Verification items for the finished model (mm, model axes). Round coordinates to 2 decimals unless told otherwise and drop trailing zeros. Loops run counter-clockwise (first coordinate to the right, second up) from the corner with the lowest first, then second, coordinate; pieces in that order, holes last. Notation, with made-up numbers: (28.25, 56) - (43.25, 56) arc R28 cw to (43.25, 82) - close; hole circle Ø1 at (47, 82.25). An arc over 180 degrees is marked (long way). Use a Markdown table: item, result. Add a question column.
```python
from build123d import *

# Parameters (mm, degrees)
SKETCH1_R                = 15
SKETCH1_R_2              = 5
BOSS_EXTRUDE1_DEPTH      = 3.2
SKETCH2_R                = 55
SKETCH2_R_2              = 45
BOSS_EXTRUDE2_DEPTH      = 3.2
BOSS_EXTRUDE3_DEPTH      = 3.2
SKETCH3_R                = 1.75
CUT_EXTRUDE2_DEPTH       = 4.2
SKETCH4_R                = 2.75
CUT_EXTRUDE3_DEPTH       = 4.2
FILLET1_R                = 4
CIRPATTERN1_COUNT        = 6
FILLET1_OF_CIRPATTERN1_R = 4
CIRPATTERN2_COUNT        = 6


with BuildPart() as part:
    # Sketch1 → Boss-Extrude1 (new body)
    with BuildSketch(Plane(origin=(0, 0, 0), x_dir=(1, 0, 0), z_dir=(0, 1, 0))):
        Circle(SKETCH1_R)
        Circle(SKETCH1_R_2, mode=Mode.SUBTRACT)
    extrude(amount=BOSS_EXTRUDE1_DEPTH)



with BuildPart() as body_2:
    # Sketch2 → Boss-Extrude2 (new body)
    with BuildSketch(Plane(origin=(0, 0, 0), x_dir=(1, 0, 0), z_dir=(0, 1, 0))):
        Circle(SKETCH2_R)
        Circle(SKETCH2_R_2, mode=Mode.SUBTRACT)
    extrude(amount=BOSS_EXTRUDE2_DEPTH)


with BuildPart() as part_1:
    add(part.part)

    add(body_2.part)  # Boss-Extrude3 merges body 2
    # Sketch5 → Boss-Extrude3 (add)
    with BuildSketch(Plane(origin=(0, 0, 0), x_dir=(1, 0, 0), z_dir=(0, 1, 0))):
        with BuildLine():
            Line((-5.098732434, 44.710210552), (-3, 14.696938457))
            ThreePointArc((-3, 14.696938457), (0, 15), (3, 14.696938457))
            Line((3, 14.696938457), (5.098732434, 44.710210552))
            ThreePointArc((5.098732434, 44.710210552), (0, 45), (-5.098732434, 44.710210552))
        make_face()
    boss_extrude3 = extrude(amount=BOSS_EXTRUDE3_DEPTH)

    # Sketch3 → Cut-Extrude2 (cut, through all)
    with BuildSketch(Plane(origin=(0, 0, 0), x_dir=(1, 0, 0), z_dir=(0, 1, 0))):
        with Locations((0, 10)):
            Circle(SKETCH3_R)
    cut_extrude2 = extrude(amount=CUT_EXTRUDE2_DEPTH, mode=Mode.SUBTRACT)

    # Sketch4 → Cut-Extrude3 (cut, through all)
    with BuildSketch(Plane(origin=(0, 0, 0), x_dir=(1, 0, 0), z_dir=(0, 1, 0))):
        with Locations((0, 50)):
            Circle(SKETCH4_R)
    cut_extrude3 = extrude(amount=CUT_EXTRUDE3_DEPTH, mode=Mode.SUBTRACT)

    # Fillet1
    fillet1_edges = [part_1.edges().sort_by_distance(p)[0] for p in [
        (5.098732434, 1.6, -44.710210552),
        (-5.098732434, 1.6, -44.710210552),
        (-3, 1.6, -14.696938457),
        (3, 1.6, -14.696938457),
    ]]
    fillet(fillet1_edges, radius=FILLET1_R)

    # CirPattern1: Boss-Extrude3, Cut-Extrude3 ×6 about axis
    cirpattern1_axis = Axis((0, 0, 0), (0, 1, 0))
    for i in range(1, CIRPATTERN1_COUNT):
        add(boss_extrude3.rotate(cirpattern1_axis, i * 360 / CIRPATTERN1_COUNT))
        add(cut_extrude3.rotate(cirpattern1_axis, i * 360 / CIRPATTERN1_COUNT), mode=Mode.SUBTRACT)

    # Fillet1 of CirPattern1
    fillet1_of_cirpattern1_edges = [part_1.edges().sort_by_distance(p)[0] for p in [
        (-36.170811929, 1.6, -26.77073709),
        (-41.269544363, 1.6, -17.939473461),
        (-14.227922061, 1.6, -4.750393017),
        (-11.227922061, 1.6, -9.94654544),
        (-41.269544363, 1.6, 17.939473461),
        (-36.170811929, 1.6, 26.77073709),
        (-11.227922061, 1.6, 9.94654544),
        (-14.227922061, 1.6, 4.750393017),
        (-5.098732434, 1.6, 44.710210552),
        (5.098732434, 1.6, 44.710210552),
        (3, 1.6, 14.696938457),
        (-3, 1.6, 14.696938457),
        (36.170811929, 1.6, 26.77073709),
        (41.269544363, 1.6, 17.939473461),
        (14.227922061, 1.6, 4.750393017),
        (11.227922061, 1.6, 9.94654544),
        (41.269544363, 1.6, -17.939473461),
        (36.170811929, 1.6, -26.77073709),
        (11.227922061, 1.6, -9.94654544),
        (14.227922061, 1.6, -4.750393017),
    ]]
    fillet(fillet1_of_cirpattern1_edges, radius=FILLET1_OF_CIRPATTERN1_R)

    # CirPattern2: Cut-Extrude2 ×6 about axis
    cirpattern2_axis = Axis((0, 0, 0), (0, 1, 0))
    for i in range(1, CIRPATTERN2_COUNT):
        add(cut_extrude2.rotate(cirpattern2_axis, i * 360 / CIRPATTERN2_COUNT), mode=Mode.SUBTRACT)


solid = part_1.part
```
Q1. Section check B-B on z = -32. Record the cut outline in (x, y), plus the area to 3 significant figures.
Q2. Section check A-A on z = 0. Record the cut outline in (x, y), plus the area to 3 significant figures.
Q3. Release check for a two-part mould opening along X. For faces 1 (the face through (-15.319, 1.622, 4.462)), 2 (the face through (40.68, 1.58, -24.17)) record: +X half, -X half, draft (parallel to the pull), parting line (faces both ways), or undercut.
Q4. Section check C-C on y = 1.9. State how many separate pieces and enclosed holes the cut face has, plus the area to 3 significant figures.
Q5. Section check D-D on z = 29. Record the cut outline in (x, y).
Q6. Go/stop test with flat-tipped pins: pin 1 Ø4.5 at (x, z) = (43.3, 25) entering from -Y; pin 2 Ø1.5 at (x, y) = (-9.5, 2.5) entering from +Z. Record where each tip stops, or that it passes through.
Q7. Thickness scan on line 1 along Z through (x, y) = (0, 0.85); line 2 along Z through (x, y) = (45.5, 1.4); line 3 along X through (y, z) = (1.95, 29). Record the ranges inside material, lowest first.
Determined:
| question | item | result |
|---|---|---|
| 1 | outline | (-44.73, 0) - (-31.64, 0) - (-31.64, 3.2) - (-44.73, 3.2) - close; (-4.21, 0) - (4.21, 0) - (4.21, 3.2) - (-4.21, 3.2) - close; (31.64, 0) - (44.73, 0) - (44.73, 3.2) - (31.64, 3.2) - close |
| 1 | area | 111 mm² |
| 2 | outline | (-55, 0) - (-45, 0) - (-45, 3.2) - (-55, 3.2) - close; (-15, 0) - (-5, 0) - (-5, 3.2) - (-15, 3.2) - close; (5, 0) - (15, 0) - (15, 3.2) - (5, 3.2) - close; (45, 0) - (55, 0) - (55, 3.2) - (45, 3.2) - close |
| 2 | area | 128 mm² |
| 3 | face 1 | undercut |
| 3 | face 2 | undercut |
| 4 | separate pieces | 1 |
| 4 | enclosed holes | 19 |
| 4 | area | 5,110 mm² |
| 5 | outline | (-46.73, 0) - (-34.05, 0) - (-34.05, 3.2) - (-46.73, 3.2) - close; (-4, 0) - (4, 0) - (4, 3.2) - (-4, 3.2) - close; (34.05, 0) - (46.73, 0) - (46.73, 3.2) - (34.05, 3.2) - close |
| 6 | pin 1 | passes through |
| 6 | pin 2 | stops at z = 54.3 |
| 7 | line 1 | z = -55 to -52.75, -47.25 to -11.75, -8.25 to -5, 5 to 8.25, 11.75 to 47.25, 52.75 to 55 |
| 7 | line 2 | z = -30.9 to -26.65, -23.35 to 23.35, 26.65 to 30.9 |
| 7 | line 3 | x = -46.73 to -34.05, -4 to 4, 34.05 to 46.73 |
